from build123d import *

# Parameters (mm, degrees)
F1_DEPTH = 16
F2_W     = 60
F2_H     = 82
F3_DEPTH = 4
F4_W     = 48
F4_H     = 82
F5_DEPTH = 4
F6_R     = 3
F7_R     = 5.5
F8_DEPTH = 20.001


with BuildPart() as f1:
    # F0 (on Top) → F1 (new body)
    with BuildSketch(Plane.XY):
        with BuildLine():
            ThreePointArc((-54, 0), (-63.899495, -4.100505), (-68, -14))
            Line((-68, -14), (-68, -68))
            ThreePointArc((-68, -68), (-63.899495, -77.899495), (-54, -82))
            Line((-54, -82), (54, -82))
            ThreePointArc((54, -82), (63.899495, -77.899495), (68, -68))
            Line((68, -68), (68, -14))
            ThreePointArc((68, -14), (63.899495, -4.100505), (54, 0))
            Line((54, 0), (-54, 0))
        make_face()
    extrude(amount=F1_DEPTH)

    # F2 (on Top) → F3 (join)
    with BuildSketch(Plane.XY):
        with Locations((0, -41)):
            Rectangle(F2_W, F2_H)
    extrude(amount=-F3_DEPTH)

    # F4 (on face) → F5 (cut)
    with BuildSketch(Plane.XY.offset(16)):
        with Locations((0, -41)):
            Rectangle(F4_W, F4_H)
    extrude(amount=-F5_DEPTH, mode=Mode.SUBTRACT)

    # F6
    f6_edges = [f1.edges().sort_by_distance(p)[0] for p in [
        (-24, -41, 12),
        (24, -41, 12),
    ]]
    fillet(f6_edges, radius=F6_R)

    # F7 (on face) → F8 (cut, through all)
    with BuildSketch(Plane.XY.offset(16)):
        with Locations((54, -14)):
            Circle(F7_R)
        with Locations((54, -68)):
            Circle(F7_R)
        with Locations((-54, -14.32929)):
            Circle(F7_R)
        with Locations((-54, -68.32929)):
            Circle(F7_R)
    extrude(amount=-F8_DEPTH, mode=Mode.SUBTRACT)


solid = f1.part
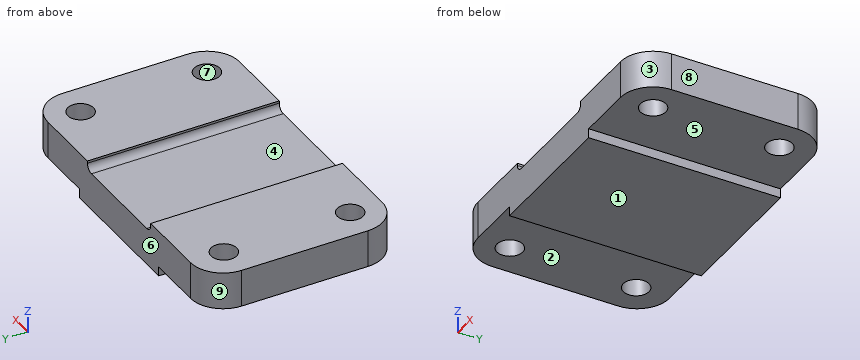
Build history of the part. All positions in model axes, mm. Face numbers are marked on the shaded views. A direction names the side the tool comes from. Give positions to 0.01 mm unless a question says otherwise; leave off trailing zeros. Order: outer loops, then holes, each group sorted by start corner. A loop starts at its lowest first (then second) coordinate and runs counter-clockwise, first axis right, second up. Notation, with made-up numbers: M 76,-8.75 L 92,-8.75 A26 cw 92,27.25 Z; hole C 67,89.25 d4. An arc over 180 degrees is marked long. Put each result on its own line as item: value.
Item 1: Pull direction X, two halves, no side cores. Call the marked faces 6, 7, 8 and 9: +X half, -X half, draft (parallel to the pull), parting line (faces both ways), or undercut.
Results are:
face 6: draft
face 7: undercut
face 8: +X half
face 9: -X half
Item 2: Cut at B-B on y = -43. Write the cut outline in (x, z), then the cut area to 3 significant figures.
Results are:
outline: M -68,0 L -30,0 L -30,-4 L 30,-4 L 30,0 L 68,0 L 68,16 L 24,16 L 24,15 A3 cw 21,12 L -21,12 A3 cw -24,15 L -24,16 L -68,16 Z
area: 2,230 mm2
Item 3: Cut at C-C on z = -2. Write the cut outline in (x, y).
Results are:
outline: M -30,-82 L 30,-82 L 30,0 L -30,0 Z
Item 4: Cut at A-A on z = 6.75. Write the cut outline in (x, y), then the cut area to 3 significant figures.
Results are:
outline: M -68,-68 A14 ccw -54,-82 L 54,-82 A14 ccw 68,-68 L 68,-14 A14 ccw 54,0 L -54,0 A14 ccw -68,-14 Z; hole C -54,-68.33 d11; hole C -54,-14.33 d11; hole C 54,-68 d11; hole C 54,-14 d11
area: 10,600 mm2
Item 5: Cut at D-D on x = 38.5. Write the cut outline in (y, z).
Results are:
outline: M -82,0 L 0,0 L 0,16 L -82,16 Z
Item 6: Wall check: probe 1 along Y at (x, z) = (-54, 11.25); probe 2 along X at (y, z) = (-14.5, 10); probe 3 along Y at (x, z) = (54, 9.25). Give the ranges that are in metal, low to high.
Results are:
probe 1: -82 to -73.83, -62.83 to -19.83, -8.83 to 0
probe 2: -68 to -59.5, -48.5 to 48.52, 59.48 to 68
probe 3: -82 to -73.5, -62.5 to -19.5, -8.5 to 0
Item 7: Which spindle directions (+Z, -Z, +X, -X, +Y, -Y) get a long thin tool onto all of the face, cutting with end or side? Do the marked faces 1, 2, 3, 4 and 5. Say none if no direction does.
Results are:
face 1: -Z, +X, -X, +Y, -Y
face 2: -Z, -X, +Y, -Y
face 3: +Z, -Z, +X, -Y
face 4: +Z, +Y, -Y
face 5: -Z, +X, +Y, -Y
Item 8: Drop flat-ended pins along their axis: pin 1 Ø17.5 at (x, y) = (54, -14) entering from -Z; pin 2 Ø12.5 at (x, y) = (-0.5, -34) entering from +Z; pin 3 Ø1.5 at (x, z) = (12.5, 10.5) entering from +Y; pin 4 Ø6.5 at (x, y) = (-54, -68.33) entering from +Z. Give the stop position or say it passes through.
Results are:
pin 1: z = 0
pin 2: z = 12
pin 3: y = 0
pin 4: through
